Input: dimensioned drawing with shaded views. Units: mm. Origin: part minimum x, y, z. Give positions to 0.01 mm unless a question says otherwise; leave off trailing zeros. Loops run counter-clockwise (first coordinate to the right, second up) from the corner with the lowest first, then second, coordinate; pieces in that order, holes last.
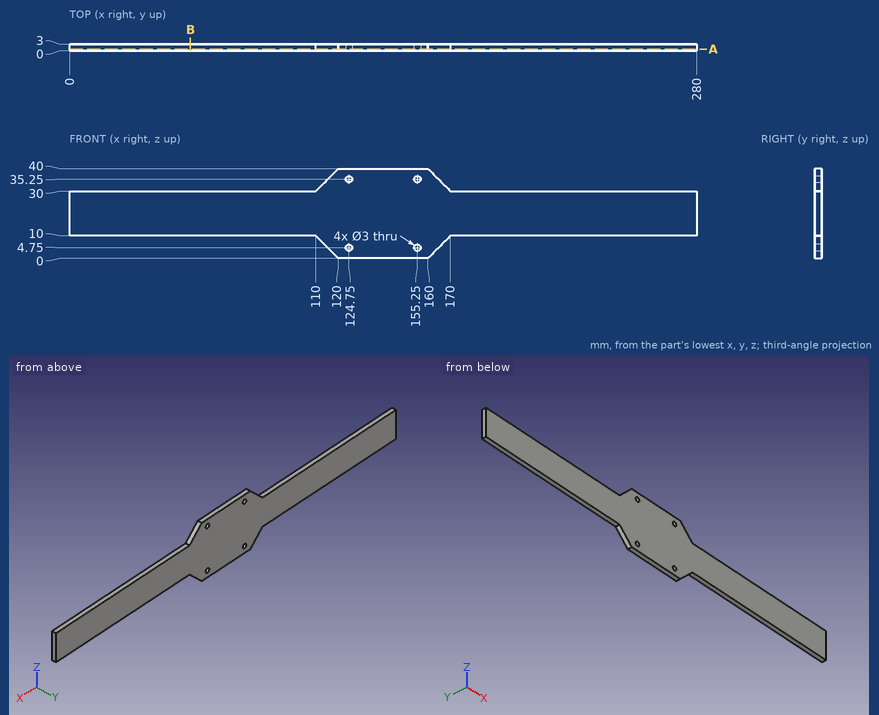
(1) First-contact query: pin 1 (1.5 mm diameter, centred on x = 29.5, y = 2.5, fed in from +Z); pin 2 (1.5 mm diameter, centred on x = 63.5, y = 2, fed in from -Z); pin 3 (3 mm diameter, centred on x = 69.5, z = 32.5, fed in from -Y). Flat tips, straight axial feed; report the tip coordinate or a pass-through.
A:
pin 1: stops at z = 30
pin 2: stops at z = 10
pin 3: passes through
(2) Ray query, line 1 along Z through (x, y) = (155.25, 2); line 2 along X through (y, z) = (1.9, 4.75); line 3 along X through (y, z) = (1.95, 35.5). Return the intervals inside material, ascending.
A:
line 1: z = 0 to 3.25, 6.25 to 33.75, 36.75 to 40
line 2: x = 115.25 to 123.25, 126.25 to 153.75, 156.75 to 164.75
line 3: x = 115.5 to 123.27, 126.23 to 153.77, 156.73 to 164.5
(3) Section B-B, the plane x = 54. Return the cut outline in (y, z), then the cut area to 3 significant figures.
A:
outline: (0, 10) - (3, 10) - (3, 30) - (0, 30) - close
area: 60.0 mm2
(4) Section A-A, the plane y = 0.75. Return the cut outline in (x, z), then the cut area to 3 significant figures.
A:
outline: (0, 10) - (110, 10) - (120, 0) - (160, 0) - (170, 10) - (280, 10) - (280, 30) - (170, 30) - (160, 40) - (120, 40) - (110, 30) - (0, 30) - close; hole circle Ø3 at (124.75, 4.75); hole circle Ø3 at (124.75, 35.25); hole circle Ø3 at (155.25, 4.75); hole circle Ø3 at (155.25, 35.25)
area: 6,570 mm2
